from build123d import *

# Parameters (mm, degrees)
SKETCH_1_R          = 2.625
SKETCH_1_R_2        = 21
EXTRUDE_1_DEPTH     = 15
EXTRUDE_START       = 6
EXTRUDE_2_DEPTH     = 6
FILLET_1_R          = 7
CHAMFER_1_SIZE      = 1
SKETCH_3_R          = 2.25
CUT_EXTRUDE_1_DEPTH = 48.335527685
CUT_EXTRUDE_2_DEPTH = 3


with BuildPart() as part:
    # Эскиз1 → Бобышка-Вытянуть1 (new body)
    with BuildSketch(Plane(origin=(0, 0, 0), x_dir=(1, 0, 0), z_dir=(0, 1, 0))):
        with BuildLine():
            ThreePointArc((25.949265582, -7.458928593), (23.382685902, 13.5), (6.515011145, 26.2021875))
            ThreePointArc((6.515011145, 26.2021875), (0, 31.625), (-6.515011145, 26.2021875))
            ThreePointArc((-6.515011145, 26.2021875), (-23.382685902, 13.5), (-25.949265582, -7.458928593))
            ThreePointArc((-25.949265582, -7.458928593), (-27.388053395, -15.8125), (-19.434254437, -18.743258907))
            ThreePointArc((-19.434254437, -18.743258907), (0, -27), (19.434254437, -18.743258907))
            ThreePointArc((19.434254437, -18.743258907), (27.388053395, -15.8125), (25.949265582, -7.458928593))
        make_face()
        with Locations(Location((0, 25, 0), (0, 0, 270))):
            Circle(SKETCH_1_R, mode=Mode.SUBTRACT)
        with Locations(Location((0, 0, 0), (0, 0, 270))):
            Circle(SKETCH_1_R_2, mode=Mode.SUBTRACT)
        with Locations(Location((-21.650635095, -12.5, 0), (0, 0, 270))):
            Circle(SKETCH_1_R, mode=Mode.SUBTRACT)
        with Locations(Location((21.650635095, -12.5, 0), (0, 0, 270))):
            Circle(SKETCH_1_R, mode=Mode.SUBTRACT)
    extrude(amount=EXTRUDE_1_DEPTH)

    # Эскиз2 → Бобышка-Вытянуть2 (add)
    with BuildSketch(Plane.XZ.offset(EXTRUDE_START)):
        with BuildLine():
            ThreePointArc((25.949265582, 7.458928593), (27.388053395, 15.8125), (19.434254437, 18.743258907))
            ThreePointArc((19.434254437, 18.743258907), (0, 27), (-19.434254437, 18.743258907))
            ThreePointArc((-19.434254437, 18.743258907), (-27.388053395, 15.8125), (-25.949265582, 7.458928593))
            ThreePointArc((-25.949265582, 7.458928593), (-23.382685902, -13.5), (-6.515011145, -26.2021875))
            ThreePointArc((-6.515011145, -26.2021875), (0, -31.625), (6.515011145, -26.2021875))
            ThreePointArc((6.515011145, -26.2021875), (23.382685902, -13.5), (25.949265582, 7.458928593))
        make_face()
    extrude(amount=-EXTRUDE_2_DEPTH)

    # Скругление1
    fillet_1_edges = [part.edges().sort_by_distance(p)[0] for p in [
        (19.434254437, 4.5, 18.743258907),
        (-19.434254437, 4.5, 18.743258907),
        (-25.949265582, 4.5, 7.458928593),
        (-6.515011145, 4.5, -26.2021875),
        (6.515011145, 4.5, -26.2021875),
        (25.949265582, 4.5, 7.458928593),
    ]]
    fillet(fillet_1_edges, radius=FILLET_1_R)

    # Фаска1
    chamfer_1_edges = [part.edges().sort_by_distance(p)[0] for p in [
        (21.650635095, 15, 9.875),
        (0, 15, -27.625),
        (-21.650635095, 15, 9.875),
    ]]
    chamfer(chamfer_1_edges, length=CHAMFER_1_SIZE)

    # Эскиз3 → Вырез-Вытянуть1 (cut, through all)
    with BuildSketch(Plane.XZ.offset(6)):
        with Locations(Location((0, 10.5, 0), (0, 0, 270))):
            Circle(SKETCH_3_R)
        with Locations(Location((9.09326674, -5.25, 0), (0, 0, 270))):
            Circle(SKETCH_3_R)
        with Locations(Location((-9.09326674, -5.25, 0), (0, 0, 270))):
            Circle(SKETCH_3_R)
    extrude(amount=-CUT_EXTRUDE_1_DEPTH, mode=Mode.SUBTRACT)

    # Эскиз4 → Вырез-Вытянуть2 (cut)
    with BuildSketch(Plane(origin=(0, 0, 0), x_dir=(1, 0, 0), z_dir=(0, 1, 0))):
        Polygon((-4.070319398, -10.5), (-2.035159699, -14.025), (2.035159699, -14.025), (4.070319398, -10.5), (2.035159699, -6.975), (-2.035159699, -6.975), align=None)
        Polygon((11.128426439, 1.725), (13.163586138, 5.25), (11.128426439, 8.775), (7.058107041, 8.775), (5.022947342, 5.25), (7.058107041, 1.725), align=None)
        Polygon((-7.058107041, 8.775), (-11.128426439, 8.775), (-13.163586138, 5.25), (-11.128426439, 1.725), (-7.058107041, 1.725), (-5.022947342, 5.25), align=None)
    extrude(amount=-CUT_EXTRUDE_2_DEPTH, mode=Mode.SUBTRACT)


solid = part.part
Source: CAD feature listing. Evaluate the final solid. Frame: model axes, mm. A direction names the side the tool comes from. Give positions to 0.01 mm unless a question says otherwise; leave off trailing zeros. Write each loop counter-clockwise with the first axis right and the second up, starting at its lowest first coordinate (ties: lowest second). Pieces come first, ordered by that corner, then holes. Notation, with made-up numbers: M 23,-19 L 32,-19 A16 cw 32,-4 Z; hole C 57.5,3.5 d1. An arc over 180 degrees is marked long. Answer as a JSON object with one key per item and string values.
Q1. Cut plane B-B, the plane z = 0. Return the cut outline in (x, y).
Geometry check:
{"outline": "M -27,-6 L 27,-6 L 27,15 L 21,15 L 21,0 L -21,0 L -21,15 L -27,15 Z"}
Q2. Cut plane A-A, the plane x = 0. Return the cut outline in (y, z) (3 decimals).
Geometry check:
{"outline": "M -6,-31.625 L 15,-31.625 L 15,-28.625 L 14,-27.625 L 0,-27.625 L 0,-22.375 L 14,-22.375 L 15,-21.375 L 15,-21 L 0,-21 L 0,6.975 L -3,6.975 L -3,8.25 L -6,8.25 Z; M -6,12.75 L -3,12.75 L -3,14.025 L 0,14.025 L 0,21 L 15,21 L 15,27 L -6,27 Z"}
Q3. Ray query, line 1 along X through (y, z) = (-3.75, -5.25); line 2 along X through (y, z) = (8, 12.5); line 3 along Y through (x, z) = (-2.5, -12). Return the intervals inside material, ascending.
Geometry check:
{"line 1": "x = -26.48 to -11.34, -6.84 to 6.84, 11.34 to 26.48", "line 2": "x = -28.28 to -24.28, -19.03 to -16.87, 16.87 to 19.03, 24.28 to 28.28", "line 3": "y = -6 to 0"}
Q4. Contact query for flat-ended pins moving along their axis: P1, Ø2, axis at x = -11, z = -5.5, coming from the +Y side; P2, Ø1.5, axis at x = -9, y = -2, coming from the -Z side; P3, Ø2.5, axis at x = 22, z = 12, coming from the +Y side; P4, Ø2.5, axis at x = 0, z = 10.5, coming from the -Y side (1 decimal). Output: stop coordinate, or through.
Geometry check:
{"P1": "stops at y = -3", "P2": "stops at z = -25.84", "P3": "stops at y = 0", "P4": "passes through"}
Q5. Cut plane C-C, the plane y = -4.5. Count the separate pieces of the cut face and the enclosed holes in it, then the cut area to 3 significant figures.
Geometry check:
{"separate pieces": "1", "enclosed holes": "3", "area": "2,390 mm^2"}
Q6. Mould query, pull axis Z, two halves, no side actions, for faces 3 (the face through (20.05, 6.9, 10.42)), 4 (the face through (-13, 15, -18)), 5 (the face through (0, 4, 27)). Classes: +Z half, -Z half, draft (parallel to the pull), parting line (faces both ways), or undercut.
Geometry check:
{"face 3": "undercut", "face 4": "draft", "face 5": "+Z half"}
Q7. Access query for faces 1 (the face through (0.099, -4.521, 12.748)), 2 (the face through (9, -1, -1.725)). Directions: +Z, -Z, +X, -X, +Y, -Y. A direction counts if a zero-diameter tool reaches every point of the face in a straight line with its end or side. Return the directions, or none.
Geometry check:
{"face 1": "+Y, -Y", "face 2": "+Y"}
